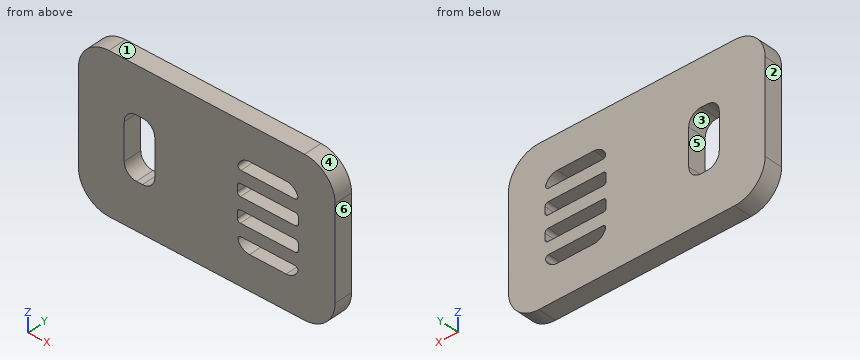
Autodesk Inventor part; units mm, degrees
ref_plane "YZ Plane" through (0, 0, 0) normal (1, 0, 0) x (0, 1, 0)
ref_plane "XZ Plane" through (0, 0, 0) normal (0, 1, 0) x (-1, 0, 0)
ref_plane "XY Plane" through (0, 0, 0) normal (0, 0, 1) x (1, 0, 0)
sketch "Sketch1" plane through (0, 0, 0) normal (0, 1, 0) x (-1, 0, 0)
  line L0 (0, -5) -> (32, -5)
  line L1 (32, 20) -> (0, 20)
  line L2 (-5, 15) -> (-5, 0)
  arc A0 (0, 20) -> (-5, 15) centre (0, 15) ccw
  arc A1 (-5, 0) -> (0, -5) centre (0, 0) ccw
  line L3 (3, 0.5) -> (9, 0.5)
  line L4 (9, 14.5) -> (3, 14.5)
  line L5 (1.5858, 12.5) -> (10.4142, 12.5)
  line L6 (1.5, 10.5) -> (10.5, 10.5)
  line L7 (1.5, 8.5) -> (10.5, 8.5)
  line L8 (1.5, 6.5) -> (10.5, 6.5)
  line L9 (1.5, 4.5) -> (10.5, 4.5)
  line L10 (1.5858, 2.5) -> (10.4142, 2.5)
  arc A2 (3, 14.5) -> (1.1144, 13.1667) centre (3, 12.5) ccw
  arc A3 (10.8856, 13.1667) -> (9, 14.5) centre (9, 12.5) ccw
  arc A4 (1.1144, 1.8333) -> (3, 0.5) centre (3, 2.5) ccw
  arc A5 (9, 0.5) -> (10.8856, 1.8333) centre (9, 2.5) ccw
  line L11 (11, 5) -> (11, 6)
  line L12 (1, 6) -> (1, 5)
  line L13 (1, 10) -> (1, 9)
  line L14 (11, 9) -> (11, 10)
  arc A6 (1.5858, 2.5) -> (1.1144, 1.8333) centre (1.5858, 2) ccw
  arc A7 (10.8856, 1.8333) -> (10.4142, 2.5) centre (10.4142, 2) ccw
  arc A8 (10.5, 4.5) -> (11, 5) centre (10.5, 5) ccw
  arc A9 (11, 6) -> (10.5, 6.5) centre (10.5, 6) ccw
  arc A10 (1.5, 6.5) -> (1, 6) centre (1.5, 6) ccw
  arc A11 (1, 5) -> (1.5, 4.5) centre (1.5, 5) ccw
  arc A12 (1, 9) -> (1.5, 8.5) centre (1.5, 9) ccw
  arc A13 (1.5, 10.5) -> (1, 10) centre (1.5, 10) ccw
  arc A14 (11, 10) -> (10.5, 10.5) centre (10.5, 10) ccw
  arc A15 (10.5, 8.5) -> (11, 9) centre (10.5, 9) ccw
  arc A16 (1.1144, 13.1667) -> (1.5858, 12.5) centre (1.5858, 13) ccw
  arc A17 (10.4142, 12.5) -> (10.8856, 13.1667) centre (10.4142, 13) ccw
  arc A18 (37, 15) -> (32, 20) centre (32, 15) ccw
  arc A19 (32, -5) -> (37, 0) centre (32, 0) ccw
  line L15 (37, 15) -> (37, 0)
  line L16 (26.5, 12.5) -> (27.5, 12.5)
  line L17 (29.5, 10.5) -> (29.5, 4.5)
  line L18 (27.5, 2.5) -> (26.5, 2.5)
  line L19 (24.5, 4.5) -> (24.5, 10.5)
  arc A20 (26.5, 12.5) -> (24.5, 10.5) centre (26.5, 10.5) ccw
  arc A21 (29.5, 10.5) -> (27.5, 12.5) centre (27.5, 10.5) ccw
  arc A22 (27.5, 2.5) -> (29.5, 4.5) centre (27.5, 4.5) ccw
  arc A23 (24.5, 4.5) -> (26.5, 2.5) centre (26.5, 4.5) ccw
  point P0 (-5, -5)
  point P1 (-5, 20)
  point P2 (37, -5)
  point P3 (24.5, 12.5)
  point P4 (29.5, 12.5)
  dimension "d0" = 42
  dimension "d2" = 25
  dimension "d3" = 5
  dimension "d4" = 5
  dimension "d5" = 5
  dimension "d8" = 5.5
  dimension "d10" = 2
  dimension "d15" = 2
  dimension "d16" = 2
  dimension "d17" = 2
  dimension "d18" = 2
  dimension "d19" = 2
  dimension "d21" = 2
  dimension "d23" = 0.5
  dimension "d30" = 2
  dimension "d31" = 6
  dimension "d32" = 16
  dimension "d37" = 5
  dimension "d41" = 5
  dimension "d42" = 42
  dimension "d43" = 7.5
  dimension "d44" = 10
  dimension "d45" = 7.5
  dimension "d46" = 2
  dimension "d49" = 5
extrude "Extrusion2" add sketch "Sketch1" along normal blind 3
properties part number "Top Block2"
Check sheet for the modelled part. Datum: model origin and axes. Units: mm. Face numbers are marked on the shaded views. A direction names the side the tool comes from. Give positions to 0.01 mm unless a question says otherwise; leave off trailing zeros. Order: outer loops, then holes, each group sorted by start corner. A loop starts at its lowest first (then second) coordinate and runs counter-clockwise, first axis right, second up. Notation, with made-up numbers: (-28, -28.75) - (-18, -28.75) arc R22 cw to (-18, -7.75) - close; hole circle Ø6 at (-21.5, 87). An arc over 180 degrees is marked (long way). Answer as CSV lines item,"result".
1. Section check C-C (x = -28). Record the boundary of the cut face in (y, z).
Result sheet:
outline,"(0, -5) - (3, -5) - (3, 2.56) - (0, 2.56) - close; (0, 12.44) - (3, 12.44) - (3, 20) - (0, 20) - close"
2. Tool access check on the marked faces 5 and 6. Record the directions out of +Z, -Z, +X, -X, +Y, -Y that give a thin tool (end or side, any length) a straight path to the whole face; none if there is none.
Result sheet:
face 5,"+Y, -Y"
face 6,"+Z, -Z, +X, +Y, -Y"
3. Section check D-D (y = 1.75). State how many separate pieces and enclosed holes the cut face has, then the cut area to 3 significant figures.
Result sheet:
separate pieces,"1"
enclosed holes,"5"
area,"906 mm²"
4. Scan lines: probe 1 along Z at (x, y) = (-27.5, 2.7); probe 2 along X at (y, z) = (1.5, 7.25); probe 3 along Z at (x, y) = (-1.5, 1.4). Record each from-to range of solid material in increasing order. Write a range as from..to.
Result sheet:
probe 1,"-5..2.5, 12.5..20"
probe 2,"-37..-29.5, -24.5..5"
probe 3,"-5..1.18, 2.49..4.5, 6.5..8.5, 10.5..12.51, 13.82..20"
5. Section check A-A (x = -4). Record the boundary of the cut face in (y, z), then the cut area to 3 significant figures.
Result sheet:
outline,"(0, -5) - (3, -5) - (3, 0.5) - (0, 0.5) - close; (0, 2.5) - (3, 2.5) - (3, 4.5) - (0, 4.5) - close; (0, 6.5) - (3, 6.5) - (3, 8.5) - (0, 8.5) - close; (0, 10.5) - (3, 10.5) - (3, 12.5) - (0, 12.5) - close; (0, 14.5) - (3, 14.5) - (3, 20) - (0, 20) - close"
area,"51.0 mm²"
6. Section check B-B (z = 7.75). Record the boundary of the cut face in (x, y).
Result sheet:
outline,"(-37, 0) - (-29.5, 0) - (-29.5, 3) - (-37, 3) - close; (-24.5, 0) - (5, 0) - (5, 3) - (-24.5, 3) - close"
7. Mould release check, pull along X, two halves, no side actions. Record for the marked faces 1, 2, 3 and 4: released by +X, released by -X, zero draft, split by the parting line, or undercut.
Result sheet:
face 1,"zero draft"
face 2,"released by -X"
face 3,"undercut"
face 4,"released by +X"
